from build123d import *

# Parameters (mm, degrees)
F0_W     = 20
F0_H     = 20
F1_DEPTH = 10
F2_R     = 3
F4_DEPTH = 1
F6_DEPTH = 1
F8_DEPTH = 1


with BuildPart() as f1:
    # F0 (on Front) → F1 (new body, symmetric)
    with BuildSketch(Plane.XZ):
        Rectangle(F0_W, F0_H)
    extrude(amount=F1_DEPTH, both=True)

    # F2
    f2_edges = [f1.edges().sort_by_distance(p)[0] for p in [
        (0, -10, 10),
        (10, 0, 10),
        (10, 0, -10),
        (10, 10, 0),
        (10, -10, 0),
        (0, -10, -10),
        (-10, -10, 0),
        (-10, 0, -10),
        (-10, 10, 0),
        (-10, 0, 10),
        (0, 10, 10),
        (0, 10, -10),
    ]]
    fillet(f2_edges, radius=F2_R)

    # F3 (on face) → F4 (cut)
    with BuildSketch(Plane.XZ.offset(10)):
        Polygon((1.5514445915, 3.9282802226), (0, 6.5010534599), (-1.5514445915, 3.9282802226), (-4.4677069853, 4.6504686339), (-3.745518574, 1.73420624), (-6.3182918114, 0.1827616486), (-3.745518574, -1.3686829429), (-4.4677069853, -4.2849453368), (-1.5514445915, -3.5627569255), (0, -6.1355301628), (1.5514445915, -3.5627569255), (4.4677069853, -4.2849453368), (3.745518574, -1.3686829429), (6.3182918114, 0.1827616486), (3.745518574, 1.73420624), (4.4677069853, 4.6504686339), align=None)
    extrude(amount=-F4_DEPTH, mode=Mode.SUBTRACT)

    # F5 (on face) → F6 (cut)
    with BuildSketch(Plane.YZ.offset(10)):
        with BuildLine():
            ThreePointArc((-0.3972897799, 4.0106111269), (-4.2636044951, 2.1552068742), (-5.7970421051, -1.849725524))
            ThreePointArc((-5.7970421051, -1.849725524), (-5.3918043168, -2.2444182335), (-4.9971116073, -1.8391804452))
            ThreePointArc((-4.9971116073, -1.8391804452), (-3.6938417401, 1.5928485864), (-0.3972897799, 3.2084230334))
            Line((-0.3972897799, 3.2084230334), (-0.3972897799, 4.0106111269))
        make_face()
        with BuildLine():
            Line((-0.3972897799, 4.7692186199), (-0.3972897799, 4.0106111269))
            ThreePointArc((-0.3972897799, 4.0106111269), (0.0027166939, 4.0242390941), (0.4027102201, 4.0102362518))
            Line((0.4027102201, 4.0102362518), (0.4027102201, 4.7692186199))
            Line((0.4027102201, 4.7692186199), (-0.3972897799, 4.7692186199))
        make_face()
        with BuildLine():
            ThreePointArc((0.4027102201, 4.0102362518), (0.0027166939, 4.0242390941), (-0.3972897799, 4.0106111269))
            Line((-0.3972897799, 4.0106111269), (-0.3972897799, 3.2084230334))
            ThreePointArc((-0.3972897799, 3.2084230334), (0.0027189433, 3.224238991), (0.4027102201, 3.2079877888))
            Line((0.4027102201, 3.2079877888), (0.4027102201, 4.0102362518))
        make_face()
        with BuildLine():
            ThreePointArc((5.7975457828, -1.7733060522), (4.2394733188, 2.1812360304), (0.4027102201, 4.0102362518))
            Line((0.4027102201, 4.0102362518), (0.4027102201, 3.2079877888))
            ThreePointArc((0.4027102201, 3.2079877888), (3.6734198381, 1.6151228676), (4.9975457828, -1.7733060522))
            ThreePointArc((4.9975457828, -1.7733060522), (5.3975457828, -2.1733060522), (5.7975457828, -1.7733060522))
        make_face()
        Polygon((-0.7970554871, 4.7692186199), (-0.3972897799, 4.7692186199), (0.4027102201, 4.7692186199), (0.7970554871, 4.7692186199), (0, 6.718759425), align=None)
        with BuildLine():
            ThreePointArc((0.4027102201, 3.2079877888), (0.0027189433, 3.224238991), (-0.3972897799, 3.2084230334))
            Line((-0.3972897799, 3.2084230334), (-0.3972897799, -4.5119822188))
            Line((-0.3972897799, -4.5119822188), (0, -3.7174872123))
            Line((0, -3.7174872123), (0.4027102201, -4.5496343811))
            Line((0.4027102201, -4.5496343811), (0.4027102201, 3.2079877888))
        make_face()
        Polygon((0, -3.7174872123), (-0.3972897799, -4.5119822188), (-0.6620978093, -5.0415419197), (-0.2579830259, -5.0415419197), (0, -4.4945096597), (0.2579830259, -5.0415419197), (0.6407644978, -5.0415419197), (0.4027102201, -4.5496343811), align=None)
        Polygon((0.2579830259, -5.0415419197), (-0.2579830259, -5.0415419197), (-0.6514311535, -5.8758170344), (0.6514311535, -5.8758170344), align=None)
        Polygon((0, -4.4945096597), (-0.2579830259, -5.0415419197), (0.2579830259, -5.0415419197), align=None)
    extrude(amount=-F6_DEPTH, mode=Mode.SUBTRACT)

    # F7 (on face) → F8 (cut)
    with BuildSketch(Plane.XY.offset(10)):
        with BuildLine():
            add(Edge.make_bspline(
                [(-5.4, 5.4), (-4.435118036, 5.0849730425), (-0.0419186137, 0.6489528576), (2.7372583002, -1.8887301628)],
                knots=[0, 0, 0, 0, 10.9243105059, 10.9243105059, 10.9243105059, 10.9243105059], degree=3))
            Line((-5.4, 5.4), (2.3129942315, -2.3129942315))
            Line((2.3129942315, -2.3129942315), (2.7372583002, -1.8887301628))
        make_face()
        with BuildLine():
            Line((2.3129942315, -2.3129942315), (-5.4, 5.4))
            add(Edge.make_bspline(
                [(-5.4, 5.4), (-5.0849730425, 4.435118036), (-0.6489528576, 0.0419186137), (1.8887301628, -2.7372583002)],
                knots=[0, 0, 0, 0, 10.9243105059, 10.9243105059, 10.9243105059, 10.9243105059], degree=3))
            Line((1.8887301628, -2.7372583002), (2.3129942315, -2.3129942315))
        make_face()
        Polygon((2.7372583002, -1.8887301628), (2.3129942315, -2.3129942315), (2.8786796564, -2.8786796564), (3.3029437252, -2.4544155877), (4.5757359313, -1.1816233816), (3.9882933746, -0.6376950884), align=None)
        Polygon((2.8786796564, -2.8786796564), (2.3129942315, -2.3129942315), (1.8887301628, -2.7372583002), (0.5941808249, -4.0318076381), (1.1816233816, -4.5757359313), (2.4544155877, -3.3029437252), align=None)
        with BuildLine():
            Line((3.3029437252, -2.4544155877), (2.8786796564, -2.8786796564))
            Line((2.8786796564, -2.8786796564), (4.2928932188, -4.2928932188))
            ThreePointArc((4.2928932188, -4.2928932188), (4.5527864045, -4.105572809), (4.8585786438, -4.0100505063))
            Line((4.8585786438, -4.0100505063), (3.3029437252, -2.4544155877))
        make_face()
        with BuildLine():
            Line((4.2928932188, -4.2928932188), (2.8786796564, -2.8786796564))
            Line((2.8786796564, -2.8786796564), (2.4544155877, -3.3029437252))
            Line((2.4544155877, -3.3029437252), (4.0100505063, -4.8585786438))
            ThreePointArc((4.0100505063, -4.8585786438), (4.105572809, -4.5527864045), (4.2928932188, -4.2928932188))
        make_face()
        with BuildLine():
            ThreePointArc((4.8585786438, -4.0100505063), (4.5527864045, -4.105572809), (4.2928932188, -4.2928932188))
            Line((4.2928932188, -4.2928932188), (4.4343145751, -4.4343145751))
            Line((4.4343145751, -4.4343145751), (4.8585786438, -4.0100505063))
        make_face()
        with BuildLine():
            Line((4.4343145751, -4.4343145751), (4.2928932188, -4.2928932188))
            ThreePointArc((4.2928932188, -4.2928932188), (4.105572809, -4.5527864045), (4.0100505063, -4.8585786438))
            Line((4.0100505063, -4.8585786438), (4.4343145751, -4.4343145751))
        make_face()
        with BuildLine():
            Line((4.8585786438, -4.0100505063), (4.4343145751, -4.4343145751))
            Line((4.4343145751, -4.4343145751), (4.0100505063, -4.8585786438))
            ThreePointArc((4.0100505063, -4.8585786438), (4.9291109799, -5.9974842088), (6, -5))
            ThreePointArc((6, -5), (5.6552017414, -4.244546045), (4.8585786438, -4.0100505063))
        make_face()
    extrude(amount=-F8_DEPTH, mode=Mode.SUBTRACT)


solid = f1.part
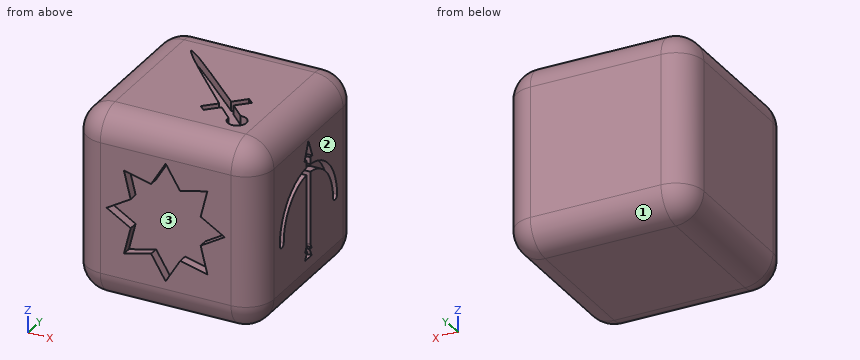
Verification items for the finished model (mm, model axes). Face numbers are marked on the shaded views. Coordinates: 2 decimals unless noted, no trailing zeros. Order: outer loops, then holes, each group sorted by start corner. A loop starts at its lowest first (then second) coordinate and runs counter-clockwise, first axis right, second up. Notation, with made-up numbers: (51, 26.5) -> (100, 26.5) arc R31 ccw to (100, 63.5) -> close; hole circle Ø1 at (75, 41.25). An arc over 180 degrees is marked (long way). Use CSV: the item, a comma, the result in double quotes. Start each with the question number.
Q1. Thickness scan on line 1 along Y through (x, z) = (1.5, 2.25); line 2 along X through (y, z) = (0, -3.5); line 3 along Z through (x, y) = (-2, 7.75). Record the ranges inside material, lowest first.
Q2. Section check A-A, the plane x = 5.25. Record the cut outline in (y, z).
Q3. Depth check by flat-ended pin: P1, Ø1.1, axis at x = 9.5, y = 0, coming from the +Z side; P2, Ø0.8, axis at x = 9.5, z = 1, coming from the -Y side; P3, Ø0.5, axis at x = 9.5, z = -2.5, coming from the +Y side. Enter the tip coordinate at first touch or a pass-through.
Q4. Draft check along Z on the marked faces 1, 2 and 3. Enter one of: +Z half, -Z half, draft (parallel to the pull), parting line (faces both ways), or undercut.
Returned:
1,line 1,"y = -9 to 10"
1,line 2,"x = -10 to 9"
1,line 3,"z = -9.9 to 9.9"
2,outline,"(-10, -7) arc R3 ccw to (-7, -10) -> (7, -10) arc R3 ccw to (10, -7) -> (10, 7) arc R3 ccw to (7, 10) -> (-4.03, 10) -> (-4.03, 9) -> (-5.97, 9) -> (-5.97, 10) -> (-7, 10) arc R3 ccw to (-10, 7) -> (-10, 0.83) -> (-9, 0.83) -> (-9, -0.46) -> (-10, -0.46) -> close"
3,P1,"stops at z = 9.28"
3,P2,"stops at y = -9.14"
3,P3,"stops at y = 8.98"
4,face 1,"-Z half"
4,face 2,"draft"
4,face 3,"undercut"
